```python
from build123d import *

# Parameters (mm, degrees)
SM_BASE_FLANGE_1_DEPTH           = 1
SM_EDGE_FLANGE_1_STRIP_W         = 5.4732
SM_EDGE_FLANGE_1_STRIP_H         = 1
SM_EDGE_FLANGE_1_STRIP_CUT_DEPTH = 139.1
SM_EDGE_FLANGE_1_DEPTH           = 139.1
SKETCH_7_R                       = 1
CUT_EXTRUDE_1_DEPTH              = 2
SKETCH_8_R                       = 1
CUT_EXTRUDE_2_DEPTH              = 2
SKETCH_9_R                       = 1
CUT_EXTRUDE_3_DEPTH              = 10
SKETCH_10_R                      = 1
CUT_EXTRUDE_4_DEPTH              = 10
SKETCH_11_R                      = 1
CUT_EXTRUDE_5_DEPTH              = 81.928131697
SKETCH_12_R                      = 1
CUT_EXTRUDE_6_DEPTH              = 10


# Sheet-metal steps are written as plain solids
with BuildPart() as part:
    # Sketch 1 → 基材-凸緣1 (new body)
    with BuildSketch(Plane.XY):
        Polygon((-69.55, 38.6), (69.55, 38.6), (69.55, 28.5), (51.5, -20), (-51.5, -20), (-69.55, 28.5), align=None)
    extrude(amount=-SM_BASE_FLANGE_1_DEPTH)

    # 邊線-凸緣1 strip (across the edge) → 邊線-凸緣1 strip cut (cut)
    with BuildSketch(Plane(origin=(-69.55, 38.6, -1), x_dir=(0, -1, 0), z_dir=(1, 0, 0))):
        with Locations((-2, -0.5)):
            Rectangle(SM_EDGE_FLANGE_1_STRIP_W, SM_EDGE_FLANGE_1_STRIP_H)
    extrude(amount=SM_EDGE_FLANGE_1_STRIP_CUT_DEPTH, mode=Mode.SUBTRACT)

    # 邊線-凸緣1 section (across the edge) → 邊線-凸緣1 (add)
    with BuildSketch(Plane(origin=(-69.55, 38.6, -1), x_dir=(0, -1, 0), z_dir=(1, 0, 0))):
        with BuildLine():
            Line((-1, 0.7366), (-1, 11))
            Line((-1, 11), (0, 11))
            Line((0, 11), (0, 0.7366))
            ThreePointArc((0, 0.7366), (0.215745145, 0.215745145), (0.7366, 0))
            Line((0.7366, 0), (0.7366, -1))
            ThreePointArc((0.7366, -1), (-0.491361636, -0.491361636), (-1, 0.7366))
        make_face()
    extrude(amount=SM_EDGE_FLANGE_1_DEPTH)

    # 草圖7 → 除料-伸長1 (cut)
    with BuildSketch(Plane.XY):
        with Locations((0, 32.8634)):
            Circle(SKETCH_7_R)
        with Locations((0, -16)):
            Circle(SKETCH_7_R)
        with Locations((52, 32.8634)):
            Circle(SKETCH_7_R)
        with Locations((26, 32.8634)):
            Circle(SKETCH_7_R)
        with Locations((-52, 32.8634)):
            Circle(SKETCH_7_R)
        with Locations((-26, 32.8634)):
            Circle(SKETCH_7_R)
        with Locations((-63.021136316, 22.425192514)):
            Circle(SKETCH_7_R)
        with Locations((-51.859762821, -7.565201643)):
            Circle(SKETCH_7_R)
        with Locations((51.859762821, -7.565201643)):
            Circle(SKETCH_7_R)
        with Locations((63.021136316, 22.425192514)):
            Circle(SKETCH_7_R)
        with Locations((44, -16)):
            Circle(SKETCH_7_R)
        with Locations((-44, -16)):
            Circle(SKETCH_7_R)
    extrude(amount=-CUT_EXTRUDE_1_DEPTH, mode=Mode.SUBTRACT)

    # 草圖8 → 除料-伸長2 (cut)
    with BuildSketch(Plane(origin=(0, 39.6, 0), x_dir=(1, 0, 0), z_dir=(0, 1, 0))):
        with Locations(Location((0, 6, 0), (0, 0, 270))):
            Circle(SKETCH_8_R)
        with Locations(Location((64.55, 6, 0), (0, 0, 270))):
            Circle(SKETCH_8_R)
        with Locations(Location((-64.55, 6, 0), (0, 0, 270))):
            Circle(SKETCH_8_R)
        with Locations(Location((-32.55, 6, 0), (0, 0, 270))):
            Circle(SKETCH_8_R)
        with Locations(Location((32.55, 6, 0), (0, 0, 270))):
            Circle(SKETCH_8_R)
    extrude(amount=-CUT_EXTRUDE_2_DEPTH, mode=Mode.SUBTRACT)

    # 草圖9 → 除料-伸長3 (cut)
    with BuildSketch(Plane.XY):
        with Locations((-6, 34.6)):
            Circle(SKETCH_9_R)
        with Locations((-16.16, 34.6)):
            Circle(SKETCH_9_R)
        with Locations(Location((16.16, 34.6, 0), (0, 0, 180))):
            Circle(SKETCH_9_R)
        with Locations(Location((6, 34.6, 0), (0, 0, 180))):
            Circle(SKETCH_9_R)
    extrude(amount=-CUT_EXTRUDE_3_DEPTH, mode=Mode.SUBTRACT)

    # 草圖10 → 除料-伸長4 (cut)
    with BuildSketch(Plane.XY):
        with Locations((-20, 19.6)):
            Circle(SKETCH_10_R)
        with Locations((20, 19.6)):
            Circle(SKETCH_10_R)
        with Locations((20, -5.4)):
            Circle(SKETCH_10_R)
        with Locations((-20, -5.4)):
            Circle(SKETCH_10_R)
    extrude(amount=-CUT_EXTRUDE_4_DEPTH, mode=Mode.SUBTRACT)

    # 草圖11 → 除料-伸長5 (cut, through all)
    with BuildSketch(Plane.XY):
        with Locations((19.73, -17.69)):
            Circle(SKETCH_11_R)
        with Locations((6, -17.69)):
            Circle(SKETCH_11_R)
        with Locations(Location((-19.73, -17.69, 0), (0, 0, 180))):
            Circle(SKETCH_11_R)
        with Locations(Location((-6, -17.69, 0), (0, 0, 180))):
            Circle(SKETCH_11_R)
    extrude(amount=-CUT_EXTRUDE_5_DEPTH, mode=Mode.SUBTRACT)

    # 草圖12 → 除料-伸長6 (cut)
    with BuildSketch(Plane.XY):
        with Locations((25.73, 24.27)):
            Circle(SKETCH_12_R)
        with Locations((27.06, 8.32)):
            Circle(SKETCH_12_R)
        with Locations((28.38, -7.62)):
            Circle(SKETCH_12_R)
    cut_extrude_6 = extrude(amount=-CUT_EXTRUDE_6_DEPTH, mode=Mode.SUBTRACT)

    # 鏡射1: 除料-伸長6 across plane
    add(cut_extrude_6.mirror(Plane(origin=(0, 0, 0), x_dir=(0, 0, 1), z_dir=(1, 0, 0))), mode=Mode.SUBTRACT)


solid = part.part
```
Geometry check sheet. Reference: the model listing, model coordinates, mm. A direction names the side the tool comes from. Round coordinates to 2 decimals unless told otherwise and drop trailing zeros. Order: outer loops, then holes, each group sorted by start corner. A loop starts at its lowest first (then second) coordinate and runs counter-clockwise, first axis right, second up. Notation, with made-up numbers: (7, -21) -> (16, -21) arc R24 cw to (16, -1) -> close; hole circle Ø9 at (71, -34.5). An arc over 180 degrees is marked (long way). Return JSON: item names as keys, results as strings. Group by question number.
Q1. Gauge pin test, flat ends, axial feed: pin 1 (1 mm diameter, centred on x = 43.5, y = 28.5, fed in from -Z); pin 2 (3 mm diameter, centred on x = -32.55, z = -6, fed in from -Y). Record the tip position at first contact, or that the pin passes through.
Q2. Tool access check on faces 1 (the flat face through (1, 9, 0)), 2 (the flat face through (-1, 38.6, -7)). Record the directions out of +Z, -Z, +X, -X, +Y, -Y that give a thin tool (end or side, any length) a straight path to the whole face; none if there is none.
Q3. Section check A-A, the plane x = -39.5. Record the boundary of the cut face in (y, z).
Q4. Material ranges on probe 1 along Y at (x, z) = (-26, -0.4); probe 2 along Y at (x, z) = (-25.73, -0.6); probe 3 along Y at (x, z) = (-20, -0.4), recorded low to high. Write a range as from..to.
Q5. Section check B-B, the plane z = -9.5. Record the boundary of the cut face in (x, y), plus the area to 3 significant figures.
Q6. Section check C-C, the plane y = 15. Record the boundary of the cut face in (x, z).
Numbers:
{
 "1": {"pin 1": "z = -1", "pin 2": "y = 38.6"},
 "2": {"face 1": "+Z, +X, -X, +Y, -Y", "face 2": "-Z, +X, -X, -Y"},
 "3": {"outline": "(-20, -1) -> (37.86, -1) arc R0.74 cw to (38.6, -1.74) -> (38.6, -12) -> (39.6, -12) -> (39.6, -1.74) arc R1.74 ccw to (37.86, 0) -> (-20, 0) -> close"},
 "4": {"probe 1": "-20..23.31, 25.23..31.86, 33.86..38.97", "probe 2": "-20..23.27, 25.27..31.9, 33.83..39.18", "probe 3": "-20..-18.65, -16.73..-6.4, -4.4..18.6, 20.6..38.97"},
 "5": {"outline": "(-69.55, 38.6) -> (69.55, 38.6) -> (69.55, 39.6) -> (-69.55, 39.6) -> close", "area": "139 mm^2"},
 "6": {"outline": "(-64.53, -1) -> (64.53, -1) -> (64.53, 0) -> (-64.53, 0) -> close"}
}
